Part model, mm, in its own coordinate system. Face numbers are marked on the shaded views. Round coordinates to 2 decimals unless told otherwise and drop trailing zeros. Order: outer loops, then holes, each group sorted by start corner. A loop starts at its lowest first (then second) coordinate and runs counter-clockwise, first axis right, second up. Notation, with made-up numbers: (32.25, -35.75) - (83.25, -35.75) arc R19 ccw to (83.25, -2.75) - close; hole circle Ø1 at (-3.5, 8). An arc over 180 degrees is marked (long way). Return JSON: item names as keys, results as strings. Group by question number.
Item 1: Probe probe 1 along Y at (x, z) = (27.5, 1.2); probe 2 along Y at (x, z) = (50, 1.25); probe 3 along X at (y, z) = (45, 0.8). List the from-to ranges inside material, lowest first.
Item 2: Saw through at C-C on z = 3.75. List the corners of the cut face in (x, y), and give its area (3 significant figures).
Item 3: Drop a flat-ended pin along its axis: pin 1 (3 mm diameter, centred on x = 27.5, y = 67.5, fed in from -Z). Give the stop position or say it passes through.
Item 4: Two-plate mould, pull along Y, no slides. Class the marked faces 1 and 2: released by +Y, released by -Y, zero draft, split by the parting line, or undercut.
Item 5: Saw through at B-B on y = 45. List the corners of the cut face in (x, z), and give its area (3 significant figures).
Item 6: Saw through at A-A on x = 50. List the corners of the cut face in (y, z), and give its area (3 significant figures).
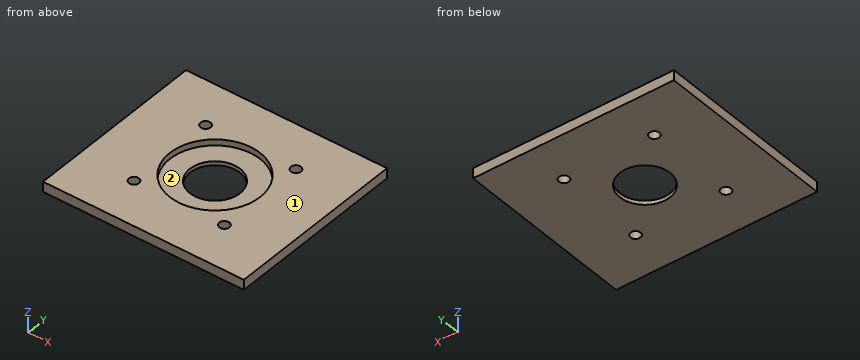
```python
from build123d import *

# Parameters (mm, degrees)
SKETCH1_W           = 100
SKETCH1_H           = 90
SKETCH1_R           = 2.5
SKETCH1_R_2         = 12.5
BOSS_EXTRUDE1_DEPTH = 5
SKETCH3_R           = 22.5
CUT_EXTRUDE2_DEPTH  = 3


with BuildPart() as part:
    # Sketch1 → Boss-Extrude1 (new body)
    with BuildSketch(Plane.XY):
        with Locations((50, 45)):
            Rectangle(SKETCH1_W, SKETCH1_H)
        with Locations((27.5, 67.5)):
            Circle(SKETCH1_R, mode=Mode.SUBTRACT)
        with Locations((72.5, 67.5)):
            Circle(SKETCH1_R, mode=Mode.SUBTRACT)
        with Locations((72.5, 22.5)):
            Circle(SKETCH1_R, mode=Mode.SUBTRACT)
        with Locations((27.5, 22.5)):
            Circle(SKETCH1_R, mode=Mode.SUBTRACT)
        with Locations((50, 45)):
            Circle(SKETCH1_R_2, mode=Mode.SUBTRACT)
    extrude(amount=BOSS_EXTRUDE1_DEPTH)

    # Sketch3 → Cut-Extrude2 (cut)
    with BuildSketch(Plane.XY.offset(5)):
        with Locations((50, 45)):
            Circle(SKETCH3_R)
    extrude(amount=-CUT_EXTRUDE2_DEPTH, mode=Mode.SUBTRACT)


solid = part.part
```
Filled in:
{
 "1": {"probe 1": "y = 0 to 20, 25 to 65, 70 to 90", "probe 2": "y = 0 to 32.5, 57.5 to 90", "probe 3": "x = 0 to 37.5, 62.5 to 100"},
 "2": {"outline": "(0, 0) - (100, 0) - (100, 90) - (0, 90) - close; hole circle Ø5 at (27.5, 22.5); hole circle Ø5 at (27.5, 67.5); hole circle Ø45 at (50, 45); hole circle Ø5 at (72.5, 22.5); hole circle Ø5 at (72.5, 67.5)", "area": "7,330 mm^2"},
 "3": {"pin 1": "passes through"},
 "4": {"face 1": "zero draft", "face 2": "undercut"},
 "5": {"outline": "(0, 0) - (37.5, 0) - (37.5, 2) - (27.5, 2) - (27.5, 5) - (0, 5) - close; (62.5, 0) - (100, 0) - (100, 5) - (72.5, 5) - (72.5, 2) - (62.5, 2) - close", "area": "315 mm^2"},
 "6": {"outline": "(0, 0) - (32.5, 0) - (32.5, 2) - (22.5, 2) - (22.5, 5) - (0, 5) - close; (57.5, 0) - (90, 0) - (90, 5) - (67.5, 5) - (67.5, 2) - (57.5, 2) - close", "area": "265 mm^2"}
}
